Read the model definition and answer for the solid it produces. Units are mm, in the model's axes. Face numbers are marked on the shaded views. A direction names the side the tool comes from. Coordinates: 2 decimals unless noted, no trailing zeros. Loops run counter-clockwise (first coordinate to the right, second up) from the corner with the lowest first, then second, coordinate; pieces in that order, holes last.
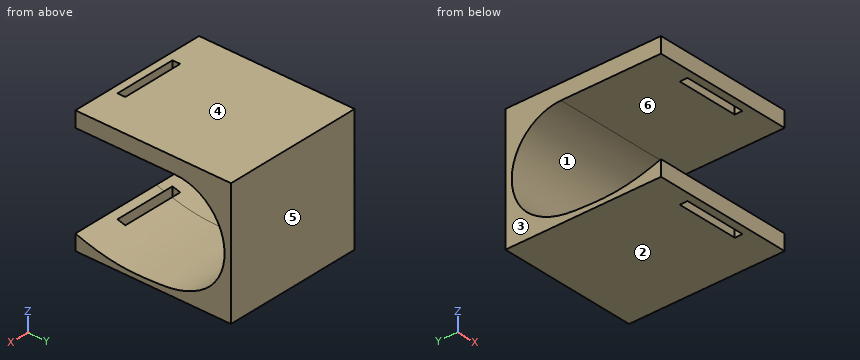
from build123d import *

# Parameters (mm, degrees)
F0_W          = 114.3
F0_H          = 101.6
F1_DEPTH      = 127
F3_DEPTH      = 39.4399856607
F3_DEPTH_BACK = 74.8620143393
F4_W          = 78.9322577574
F4_H          = 9.7147444349
F5_DEPTH      = 38.2024062272
F5_DEPTH_BACK = 63.3995939728


with BuildPart() as f1:
    # F0 (on Front) → F1 (new body)
    with BuildSketch(Plane.XZ):
        with Locations((17.7110143393, 12.5985938728)):
            Rectangle(F0_W, F0_H)
    extrude(amount=F1_DEPTH)

    # F2 (on Right) → F3 (cut, two sides)
    with BuildSketch(Plane.YZ) as f3_sk:
        with BuildLine():
            Line((-127, 50.6985938728), (-127, -25.5014061272))
            add(Edge.make_bspline(
                [(-127, -25.5014061272), (-98.9603772759, -34.7956232727), (-68.005550577, -34.5681270065), (-35.421602428, -32.3844701052), (-20.4378271917, -20.9679826113)],
                knots=[0, 0, 0, 0, 0.5357898792, 1, 1, 1, 1], degree=3))
            ThreePointArc((-20.4378271917, -20.9679826113), (-7.4607172084, 23.7360933268), (-45.4065121441, 50.6985938728))
            Line((-45.4065121441, 50.6985938728), (-127, 50.6985938728))
        make_face()
    extrude(amount=-F3_DEPTH, mode=Mode.SUBTRACT)
    extrude(f3_sk.sketch, amount=F3_DEPTH_BACK, mode=Mode.SUBTRACT)

    # F4 (on Top) → F5 (cut, two sides)
    with BuildSketch(Plane.XY) as f5_sk:
        with Locations((19.8757408652, -184.373836463)):
            Rectangle(F4_W, F4_H)
        Polygon((17.7110143393, -114.29746), (-7.6889856607, -114.29746), (-7.6889856607, -120.65), (17.7110143393, -120.65), (43.1110143393, -120.65), (43.1110143393, -114.29746), align=None)
    extrude(amount=-F5_DEPTH, mode=Mode.SUBTRACT)
    extrude(f5_sk.sketch, amount=F5_DEPTH_BACK, mode=Mode.SUBTRACT)


solid = f1.part
Item 1: A cutting plane is placed at C-C on z = 48. Determine the outline of the cut face in (x, y).
Numbers:
outline: (-39.44, -30.93) - (74.86, -30.93) - (74.86, 0) - (-39.44, 0) - close
Item 2: Which of the six approach directions +Z, -Z, +X, -X, +Y, -Y give full straight-line access (tool end or side, diameter ignored) to the marked faces 5 and 6?
Numbers:
face 5: +Z, -Z, +X, -X, +Y
face 6: +X, -X, -Y
Item 3: A cutting plane is placed at A-A on x = 34. Give the number of separate pieces and of enclosed holes in the cut face, then the cut area to 3 significant figures.
Numbers:
separate pieces: 3
enclosed holes: 0
area: 3,440 mm2
Item 4: Determine the mould class of the marked faces 1, 2, 3 and 4 for opening direction Z: released by +Z, released by -Z, zero draft, split by the parting line, or undercut.
Numbers:
face 1: undercut
face 2: released by -Z
face 3: zero draft
face 4: released by +Z
Item 5: Given pin 1 (3 mm diameter, centred on x = -18.5, z = -15.5, fed in from +Y), flat-ended and moving along its own axis, determine where the tip first touches the part or whether it passes through.
Numbers:
pin 1: stops at y = 0
Item 6: Find the intervals of material crossed by line 1 along Z through (x, y) = (-21, -33.5); line 2 along Z through (x, y) = (68, -14); line 3 along Y through (x, z) = (32.5, 4.5), in increasing order.
Numbers:
line 1: z = -38.2 to -28.52, 48.89 to 63.4
line 2: z = -38.2 to -14.55, 35.58 to 63.4
line 3: y = -5.68 to 0
Item 7: A cutting plane is placed at B-B on z = -7.5. Determine the outline of the cut face in (x, y).
Numbers:
outline: (-39.44, -9.49) - (74.86, -9.49) - (74.86, 0) - (-39.44, 0) - close
